Geometry check sheet. Reference: the model listing, model coordinates, mm. A direction names the side the tool comes from. Coordinates: 2 decimals unless noted, no trailing zeros. Order: outer loops, then holes, each group sorted by start corner. A loop starts at its lowest first (then second) coordinate and runs counter-clockwise, first axis right, second up.
```python
from build123d import *

# Parameters (mm, degrees)
BOSS_EXTRUDE1_START = 78.4
BOSS_EXTRUDE1_DEPTH = 1.6
CHAMFER1_SIZE       = 0.5
BOSS_EXTRUDE2_START = 78
BOSS_EXTRUDE2_DEPTH = 3
CHAMFER2_SIZE       = 0.5
BOSS_EXTRUDE3_START = 79.2
SKETCH3_W           = 3
SKETCH3_H           = 0.9
BOSS_EXTRUDE3_DEPTH = 0.9
BOSS_EXTRUDE4_START = -32
BOSS_EXTRUDE4_DEPTH = 4
BOSS_EXTRUDE5_START = 28
BOSS_EXTRUDE5_DEPTH = 4


with BuildPart() as part:
    # Sketch1 → Boss-Extrude1 (new body)
    with BuildSketch(Plane.XY.offset(BOSS_EXTRUDE1_START)):
        with BuildLine():
            Line((-32, 8.6), (32, 8.6))
            ThreePointArc((32, 8.6), (34.828427125, 9.771572875), (36, 12.6))
            Line((36, 12.6), (36, 30.6))
            ThreePointArc((36, 30.6), (34.828427125, 33.428427125), (32, 34.6))
            Line((32, 34.6), (-32, 34.6))
            ThreePointArc((-32, 34.6), (-34.828427125, 33.428427125), (-36, 30.6))
            Line((-36, 30.6), (-36, 12.6))
            ThreePointArc((-36, 12.6), (-34.828427125, 9.771572875), (-32, 8.6))
        make_face()
    extrude(amount=BOSS_EXTRUDE1_DEPTH)

    # Chamfer1
    chamfer1_edges = [part.edges().sort_by_distance(p)[0] for p in [
        (34.828427125, 9.771572875, 80),
        (36, 21.6, 80),
        (34.828427125, 33.428427125, 80),
        (0, 34.6, 80),
        (-34.828427125, 33.428427125, 80),
        (-36, 21.6, 80),
        (-34.828427125, 9.771572875, 80),
        (0, 8.6, 80),
    ]]
    chamfer(chamfer1_edges, length=CHAMFER1_SIZE)


with BuildPart() as body_2:
    # Sketch2 → Boss-Extrude2 (new body)
    with BuildSketch(Plane.XY.offset(BOSS_EXTRUDE2_START)):
        with BuildLine():
            Line((-3, 18.25), (3, 18.25))
            ThreePointArc((3, 18.25), (4.414213562, 18.835786438), (5, 20.25))
            Line((5, 20.25), (5, 24.25))
            ThreePointArc((5, 24.25), (4.414213562, 25.664213562), (3, 26.25))
            Line((3, 26.25), (-3, 26.25))
            ThreePointArc((-3, 26.25), (-4.414213562, 25.664213562), (-5, 24.25))
            Line((-5, 24.25), (-5, 20.25))
            ThreePointArc((-5, 20.25), (-4.414213562, 18.835786438), (-3, 18.25))
        make_face()
    extrude(amount=BOSS_EXTRUDE2_DEPTH)


with BuildPart() as part_1:
    add(part.part)

    # Combine1: cut body 2
    add(body_2.part, mode=Mode.SUBTRACT)

    # Chamfer2
    chamfer2_edges = [part_1.edges().sort_by_distance(p)[0] for p in [
        (-4.414213562, 18.835786438, 80),
        (0, 18.25, 80),
        (4.414213562, 18.835786438, 80),
        (5, 22.25, 80),
        (4.414213562, 25.664213562, 80),
        (0, 26.25, 80),
        (-4.414213562, 25.664213562, 80),
        (-5, 22.25, 80),
    ]]
    chamfer(chamfer2_edges, length=CHAMFER2_SIZE)


with BuildPart() as body_2_2:
    # Sketch3 → Boss-Extrude3 (new body)
    with BuildSketch(Plane.XY.offset(BOSS_EXTRUDE3_START)):
        with Locations((0, 8.95)):
            Rectangle(SKETCH3_W, SKETCH3_H)
    extrude(amount=BOSS_EXTRUDE3_DEPTH)


with BuildPart() as part_2:
    add(part_1.part)

    # Combine2: cut body 2 2
    add(body_2_2.part, mode=Mode.SUBTRACT)

    # Sketch4 → Boss-Extrude4 (add)
    with BuildSketch(Plane(origin=(0, 0, 0), x_dir=(0, 0, -1), z_dir=(1, 0, 0)).offset(BOSS_EXTRUDE4_START)):
        Polygon((-78.41, 12), (-74.6, 12), (-74.6, 12.8), (-74.9, 13.1), (-75.2, 13.1), (-75.2, 12.8), (-78.41, 12.8), align=None)
    extrude(amount=BOSS_EXTRUDE4_DEPTH)

    # Sketch5 → Boss-Extrude5 (add)
    with BuildSketch(Plane(origin=(0, 0, 0), x_dir=(0, 0, -1), z_dir=(1, 0, 0)).offset(BOSS_EXTRUDE5_START)):
        Polygon((-78.41, 12), (-74.6, 12), (-74.6, 12.8), (-74.9, 13.1), (-75.2, 13.1), (-75.2, 12.8), (-78.41, 12.8), align=None)
    extrude(amount=BOSS_EXTRUDE5_DEPTH)


solid = part_2.part
```
Item 1: Release check for a two-part mould opening along Y. For faces 1 (the face through (34.599, 33.142, 79.865)), 2 (the face through (34.797, 9.741, 78.942)), 3 (the face through (4.43, 25.65, 78.94)), 4 (the face through (4.4, 18.82, 78.94)) record: pulls with the +Y half, pulls with the -Y half, needs draft (parallel to the pull), parting line crosses it, or undercut.
Item 2: Sectioned sample at B-B (y = 16.25). Record the cut outline in (x, z).
Item 3: Sectioned sample at C-C (x = 27). Record the cut outline in (y, z).
Item 4: Tool access check on faces 5 (the face through (0, 16, 80)), 6 (the face through (30, 12.8, 77)), 7 (the face through (-4.4, 25.68, 78.94)), 8 (the face through (4.493, 25.776, 79.635)), 9 (the face through (-30, 12, 77)). Record the directions out of +Z, -Z, +X, -X, +Y, -Y that give a thin tool (end or side, any length) a straight path to the whole face; none if there is none.
Item 5: Sectioned sample at A-A (z = 77.55). Record the cut outline in (x, y), and give its area (3 significant figures).
Item 6: Thickness scan on line 1 along X through (y, z) = (21.25, 78.45); line 2 along Z through (x, y) = (11, 31.25); line 3 along Y through (x, z) = (28.5, 76.5). Record the ranges inside material, lowest first.
Item 7: Depth check by flat-ended pin: P1, Ø0.5, axis at y = 12.5, z = 76.5, coming from the -X side; P2, Ø1.5, axis at x = 17, y = 15.5, coming from the -Z side; P3, Ø1.2, axis at y = 12.5, z = 76, coming from the +X side. Enter the tip coordinate at first touch or a pass-through.
Geometry check:
1. face 1: pulls with the +Y half
1. face 2: pulls with the -Y half
1. face 3: undercut
1. face 4: undercut
2. outline: (-36, 78.4) - (36, 78.4) - (36, 79.5) - (35.5, 80) - (-35.5, 80) - (-36, 79.5) - close
3. outline: (8.6, 78.4) - (34.6, 78.4) - (34.6, 79.5) - (34.1, 80) - (9.1, 80) - (8.6, 79.5) - close
4. face 5: +Z, +X, -X, +Y, -Y
4. face 6: +X, -X, +Y
4. face 7: +Z, -Z
4. face 8: +Z
4. face 9: -Z, +X, -X, -Y
5. outline: (-32, 12) - (-28, 12) - (-28, 12.8) - (-32, 12.8) - close; (28, 12) - (32, 12) - (32, 12.8) - (28, 12.8) - close
5. area: 6.40 mm2
6. line 1: x = -36 to -5, 5 to 36
6. line 2: z = 78.4 to 80
6. line 3: y = 12 to 12.8
7. P1: stops at x = -32
7. P2: stops at z = 78.4
7. P3: stops at x = 32
